Geometry check sheet. Reference: drawing and pictorial views, mm from the part's lowest x, y, z. Round coordinates to 2 decimals unless told otherwise and drop trailing zeros. Loops run counter-clockwise (first coordinate to the right, second up) from the corner with the lowest first, then second, coordinate; pieces in that order, holes last. Notation, with made-up numbers: (-19, 27.5) - (7, 27.5) arc R14 cw to (7, 32.5) - close; hole circle Ø8 at (40.25, 22.5). An arc over 180 degrees is marked (long way). Answer as CSV lines item,"result". Start each with the question number.
1) Cross-section at A-A on z = 7. Record the boundary of the cut face in (x, y), and give its area (3 significant figures).
2) Cross-section at C-C on x = 6. Record the boundary of the cut face in (y, z).
3) Cross-section at B-B on y = 26. Record the boundary of the cut face in (x, z).
4) Thickness scan on line 1 along X through (y, z) = (25, 1.5); line 2 along Y through (x, z) = (26, 6); line 3 along X through (y, z) = (6.5, 3.25). Record the ranges inside material, lowest first.
5) Cross-section at D-D on z = 2. Record the boundary of the cut face in (x, y), and give its area (3 significant figures).
6) Draft check along Y on the marked faces 1, 2 and 3. Enter one of: released by +Y, released by -Y, zero draft, split by the parting line, or undercut.
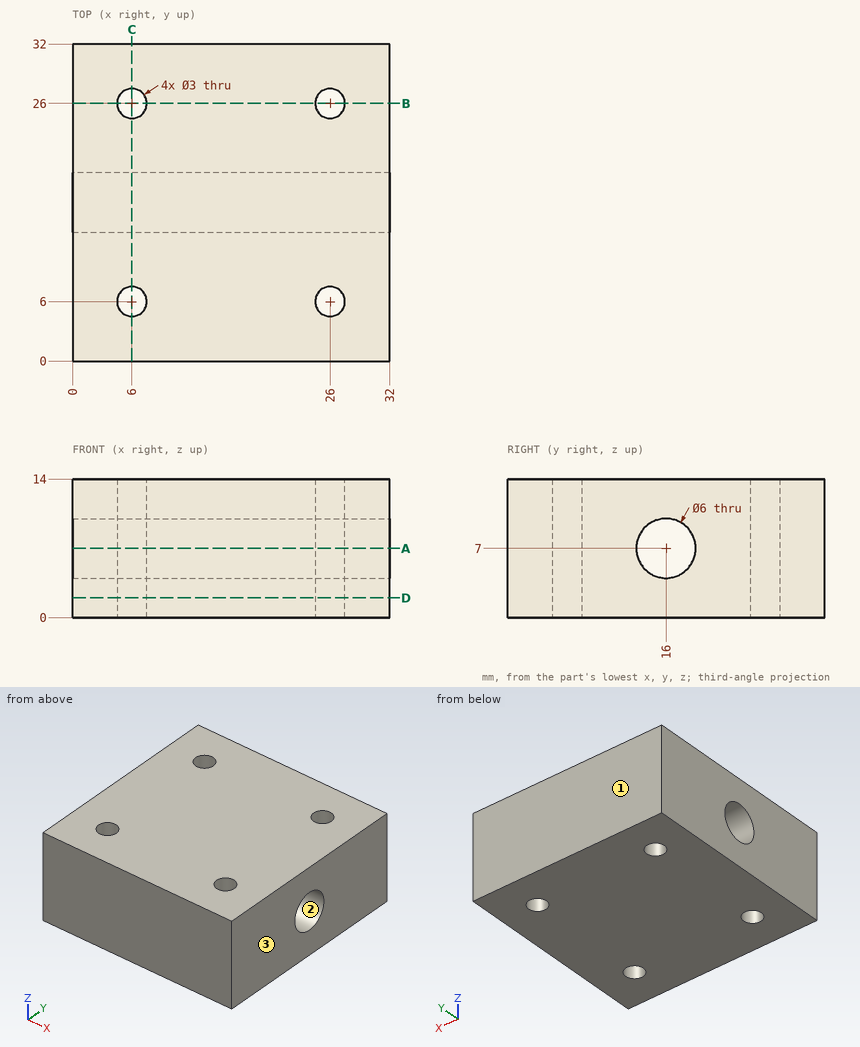
Answer block:
1,outline,"(0, 0) - (32, 0) - (32, 13) - (0, 13) - close; (0, 19) - (32, 19) - (32, 32) - (0, 32) - close; hole circle Ø3 at (6, 6); hole circle Ø3 at (6, 26); hole circle Ø3 at (26, 6); hole circle Ø3 at (26, 26)"
1,area,"804 mm^2"
2,outline,"(0, 0) - (4.5, 0) - (4.5, 14) - (0, 14) - close; (7.5, 0) - (24.5, 0) - (24.5, 14) - (7.5, 14) - close; (27.5, 0) - (32, 0) - (32, 14) - (27.5, 14) - close; hole circle Ø6 at (16, 7)"
3,outline,"(0, 0) - (4.5, 0) - (4.5, 14) - (0, 14) - close; (7.5, 0) - (24.5, 0) - (24.5, 14) - (7.5, 14) - close; (27.5, 0) - (32, 0) - (32, 14) - (27.5, 14) - close"
4,line 1,"x = 0 to 4.88, 7.12 to 24.88, 27.12 to 32"
4,line 2,"y = 0 to 4.5, 7.5 to 13.17, 18.83 to 24.5, 27.5 to 32"
4,line 3,"x = 0 to 4.59, 7.41 to 24.59, 27.41 to 32"
5,outline,"(0, 0) - (32, 0) - (32, 32) - (0, 32) - close; hole circle Ø3 at (6, 6); hole circle Ø3 at (6, 26); hole circle Ø3 at (26, 6); hole circle Ø3 at (26, 26)"
5,area,"996 mm^2"
6,face 1,"released by +Y"
6,face 2,"undercut"
6,face 3,"zero draft"
